```python
from build123d import *
from build123d.topology import SkipClean

# Parameters (mm, degrees)
SKETCH4_R           = 4.5339
SKETCH4_R_2         = 4.37515
CUT_EXTRUDE2_DEPTH  = 4.064
CUT_EXTRUDE1_DEPTH  = 4.064
CIRPATTERN1_COUNT   = 14
SKETCH6_R           = 1.5875
CUT_EXTRUDE3_DEPTH  = 12.02520933
CUT_EXTRUDE4_DEPTH  = 1.016
SKETCH9_R           = 6.985
CUT_EXTRUDE5_DEPTH  = 1.0414
SKETCH10_R          = 6.985
CUT_EXTRUDE6_DEPTH  = 6.1468
SKETCH12_R          = 1.5875
SKETCH12_R_2        = 1.4732
BOSS_EXTRUDE1_DEPTH = 3.937
BOSS_EXTRUDE2_START = 6.223
SKETCH13_R          = 3.90525
SKETCH13_R_2        = 1.4732
BOSS_EXTRUDE2_DEPTH = 6.223
BOSS_EXTRUDE3_START = 2.54
BOSS_EXTRUDE3_DEPTH = 2.54
CIRPATTERN4_COUNT   = 4


with BuildPart() as part:
    # Sketch1 → Revolve1 (revolve)
    with BuildSketch(Plane.XY, mode=Mode.PRIVATE) as revolve1_sk:
        with BuildLine():
            Line((-5.5626, 1.5875), (5.5626, 1.5875))
            Line((5.5626, 1.5875), (5.5626, 6.731))
            Line((5.5626, 6.731), (5.0419, 6.731))
            ThreePointArc((5.0419, 6.731), (4.654552953, 5.958878742), (4.5212, 5.1054))
            Line((4.5212, 5.1054), (4.5212, 4.5339))
            Line((4.5212, 4.5339), (0.4572, 4.5339))
            Line((0.4572, 4.5339), (0.4572, 5.6769))
            Line((0.4572, 5.6769), (-0.5969, 6.731))
            Line((-0.5969, 6.731), (-5.5626, 6.731))
            Line((-5.5626, 6.731), (-5.5626, 1.5875))
        make_face()
    revolve(revolve1_sk.sketch.rotate(Axis((-5.5626, 0, 0), (1, 0, 0)), 90), axis=Axis((-5.5626, 0, 0), (1, 0, 0)))

    # Sketch4 → Cut-Extrude2 (cut)
    with BuildSketch(Plane(origin=(0.4572, 0, 0), x_dir=(0, 0, -1), z_dir=(1, 0, 0))):
        Circle(SKETCH4_R)
        Circle(SKETCH4_R_2, mode=Mode.SUBTRACT)
    extrude(amount=CUT_EXTRUDE2_DEPTH, mode=Mode.SUBTRACT)

    # Sketch3 → Cut-Extrude1 (cut)
    with BuildSketch(Plane(origin=(0.4572, 0, 0), x_dir=(0, 0, -1), z_dir=(1, 0, 0))):
        with BuildLine():
            Line((-0.641613493, 4.327848154), (-0.345249615, 3.692293767))
            Line((-0.345249615, 3.692293767), (0.345249615, 3.692293767))
            Line((0.345249615, 3.692293767), (0.641613493, 4.327848154))
            ThreePointArc((0.641613493, 4.327848154), (0, 4.37515), (-0.641613493, 4.327848154))
        make_face()
    cut_extrude1 = extrude(amount=CUT_EXTRUDE1_DEPTH, mode=Mode.SUBTRACT)

    # CirPattern1: Cut-Extrude1 ×14 about axis
    cirpattern1_axis = Axis((0, 0, 0), (1, 0, 0))
    for i in range(1, CIRPATTERN1_COUNT):
        add(cut_extrude1.rotate(cirpattern1_axis, i * 360 / CIRPATTERN1_COUNT), mode=Mode.SUBTRACT)

    # Sketch6 → Cut-Extrude3 (cut, through all)
    with BuildSketch(Plane(origin=(0, 0, 0), x_dir=(1, 0, 0), z_dir=(0, 1, 0))):
        with Locations(Location((-2.5527, 0, 0), (0, 0, 90))):
            Circle(SKETCH6_R)
    extrude(amount=CUT_EXTRUDE3_DEPTH, mode=Mode.SUBTRACT)

    # Sketch9 → Cut-Extrude5 (cut)
    with BuildSketch(Plane(origin=(5.5626, 0, 0), x_dir=(0, 0, -1), z_dir=(1, 0, 0))):
        Circle(SKETCH9_R)
    extrude(amount=-CUT_EXTRUDE5_DEPTH, mode=Mode.SUBTRACT)


with BuildPart() as body_2:
    # Sketch7 → Revolve2 (revolve)
    with BuildSketch(Plane.XY, mode=Mode.PRIVATE) as revolve2_sk:
        Polygon((-3.7211, 6.731), (-2.5527, 6.731), (-2.5527, 1.9685), (-3.7211, 1.9685), (-3.9751, 2.2225), (-3.9751, 6.477), align=None)
    revolve(revolve2_sk.sketch.rotate(Axis((-2.5527, 1.9685, 0), (0, 1, 0)), 270), axis=Axis((-2.5527, 1.9685, 0), (0, 1, 0)))

    # Sketch8 → Cut-Extrude4 (cut)
    with BuildSketch(Plane(origin=(0, 6.731, 0), x_dir=(1, 0, 0), z_dir=(0, 1, 0))):
        Polygon((-2.5527, 0.821223023), (-3.2639, 0.410611511), (-3.2639, -0.410611511), (-2.5527, -0.821223023), (-1.8415, -0.410611511), (-1.8415, 0.410611511), align=None)
    extrude(amount=-CUT_EXTRUDE4_DEPTH, mode=Mode.SUBTRACT)


with BuildPart() as cut_extrude6_tool:
    # Sketch10 → Cut-Extrude6 (new body)
    with BuildSketch(Plane.ZY.offset(5.5626)):
        Circle(SKETCH10_R)
    extrude(amount=-CUT_EXTRUDE6_DEPTH)


with BuildPart() as part_1:
    add(part.part)

    # Cut-Extrude6: cut by cut_extrude6_tool
    add(cut_extrude6_tool.part, mode=Mode.SUBTRACT)

    # Sketch12 → Boss-Extrude1 (add)
    with BuildSketch(Plane(origin=(4.5212, 0, 0), x_dir=(0, 0, -1), z_dir=(1, 0, 0))):
        Circle(SKETCH12_R)
        Circle(SKETCH12_R_2, mode=Mode.SUBTRACT)
    extrude(amount=-BOSS_EXTRUDE1_DEPTH)

    # Sketch13 → Boss-Extrude2 (add)
    with BuildSketch(Plane(origin=(4.5212, 0, 0), x_dir=(0, 0, -1), z_dir=(1, 0, 0)).offset(BOSS_EXTRUDE2_START)):
        with Locations(Location((0, 0, 0), (0, 0, 186.486751227))):
            Circle(SKETCH13_R)
        Circle(SKETCH13_R_2, mode=Mode.SUBTRACT)
    extrude(amount=-BOSS_EXTRUDE2_DEPTH)

    # Sketch14 → Boss-Extrude3 (add)
    with SkipClean():  # the faces are left unmerged after this step: merging them gives an invalid solid
        with BuildSketch(Plane(origin=(10.7442, 0, 0), x_dir=(0, 0, -1), z_dir=(1, 0, 0)).offset(BOSS_EXTRUDE3_START)):
            with BuildLine():
                Line((1.361059327, -0.563769233), (3.607980544, -1.494474474))
                ThreePointArc((3.607980544, -1.494474474), (3.90525, 0), (3.607980544, 1.494474474))
                Line((3.607980544, 1.494474474), (1.361059327, 0.563769233))
                ThreePointArc((1.361059327, 0.563769233), (1.4732, 0), (1.361059327, -0.563769233))
            make_face()
        boss_extrude3 = extrude(amount=-BOSS_EXTRUDE3_DEPTH)

    # CirPattern4: Boss-Extrude3 ×4 about axis
    with SkipClean():  # the faces are left unmerged after this step: merging them gives an invalid solid
        cirpattern4_axis = Axis((-3.905928061, 0, 0), (1, 0, 0))
        for i in range(1, CIRPATTERN4_COUNT):
            add(boss_extrude3.rotate(cirpattern4_axis, i * 360 / CIRPATTERN4_COUNT))


with BuildPart() as body_2_1:
    add(body_2.part)

    # Cut-Extrude6: cut by cut_extrude6_tool
    add(cut_extrude6_tool.part, mode=Mode.SUBTRACT)


solid = part_1.part
```
Here's how the part is built. I have some questions about the finished solid (model axes, mm). A direction names the side the tool comes from. Coordinates: 2 decimals unless noted, no trailing zeros. Loops run counter-clockwise (first coordinate to the right, second up) from the corner with the lowest first, then second, coordinate; pieces in that order, holes last. Notation, with made-up numbers: (-23, 83) -> (18, 83) arc R25 ccw to (18, 117) -> close; hole circle Ø8 at (57, -22). An arc over 180 degrees is marked (long way). Return JSON: item names as keys, results as strings.
1) If we section it at C-C, the plane x = 8.25: Write out the boundary of the cut face in (y, z), then the cut area to 3 significant figures.
Results below:
{"outline": "circle Ø7.81 at (0, 0); hole circle Ø2.95 at (0, 0)", "area": "41.1 mm²"}
2) Will these pins go through, and if not, where does the flat tip stop? pin 1 (0.6 mm diameter, centred on x = 3.5, z = 0, fed in from -Y); pin 2 (0.6 mm diameter, centred on x = 3, z = 0, fed in from +Y); pin 3 (5 mm diameter, centred on x = 12, z = -3.5, fed in from -Y).
Results below:
{"pin 1": "y = -3.69", "pin 2": "y = 3.69", "pin 3": "y = -3.78"}
3) If we section it at B-B, the plane y = 0: Write out the boundary of the cut face in (x, z), then the cut area to 3 significant figures.
Results below:
{"outline": "(0.58, -4.38) -> (4.52, -4.38) -> (4.52, -3.91) -> (13.28, -3.91) -> (13.28, -1.47) -> (0.58, -1.47) -> close; (0.58, 1.47) -> (13.28, 1.47) -> (13.28, 3.91) -> (4.52, 3.91) -> (4.52, 4.38) -> (0.58, 4.38) -> close", "area": "65.5 mm²"}
4) If we section it at A-A, the plane z = 0: Write out the boundary of the cut face in (x, y).
Results below:
{"outline": "(0.58, -3.69) -> (4.52, -3.69) -> (4.52, -3.91) -> (13.28, -3.91) -> (13.28, -1.47) -> (0.58, -1.47) -> close; (0.58, 1.47) -> (13.28, 1.47) -> (13.28, 3.91) -> (4.52, 3.91) -> (4.52, 3.69) -> (0.58, 3.69) -> close"}
5) For faces 3 (the face through (4.521, 3.2, 2.5)), 4 (the face through (13.284, -3, 0)), 5 (the face through (4.521, 3.2, -2.6)), 6 (the face through (10.744, 2, -2)), 7 (the face through (4.521, -3.2, -2.6)), which set-ups out of +Z, -Z, +X, -X, +Y, -Y let a thin tool reach every point of the face, with its end or its side?
Results below:
{"face 3": "+Z, +X, +Y", "face 4": "+Z, -Z, +X, +Y, -Y", "face 5": "-Z, +X, +Y", "face 6": "+X", "face 7": "-Z, +X, -Y"}
6) I need wall thicknesses on line 1 (Z direction, x = 9, y = 0); line 2 (Y direction, x = 1.25, z = -2.75). Which ranges of each line are inside material? Lowest first, please. Write a range as from..to.
Results below:
{"line 1": "-3.91..-1.47, 1.47..3.91", "line 2": "-3.4..-2.73, -2.47..2.47, 2.73..3.4"}
7) If we section it at D-D, the plane z = 2.25: Write out the boundary of the cut face in (x, y), then the cut area to 3 significant figures.
Results below:
{"outline": "(0.58, -3.45) -> (4.52, -3.45) -> (4.52, -3.19) -> (10.74, -3.19) -> (10.74, -0.93) -> (13.28, -0.93) -> (13.28, 0.93) -> (10.74, 0.93) -> (10.74, 3.19) -> (4.52, 3.19) -> (4.52, 3.45) -> (0.58, 3.45) -> close", "area": "71.6 mm²"}
8) Thinking about a two-plate mould opening in Z: for faces 1 (the face through (10.744, 2, 2)), 2 (the face through (13.284, 3, 0)), which applies, +Z half, -Z half, draft (parallel to the pull), parting line (faces both ways), or undercut?
Results below:
{"face 1": "undercut", "face 2": "draft"}
